Could you check a few things on this model? Use its own coordinates, in mm. Face numbers are marked on the shaded views. A direction names the side the tool comes from. Round coordinates to 2 decimals unless told otherwise and drop trailing zeros. Write each loop counter-clockwise with the first axis right and the second up, starting at its lowest first coordinate (ties: lowest second). Pieces come first, ordered by that corner, then holes. Notation, with made-up numbers: (41, 13.5) - (86, 13.5) arc R7 ccw to (86, 22.5) - close; hole circle Ø9 at (36.25, -29.75). An arc over 180 degrees is marked (long way). Put each result on its own line as item: value.
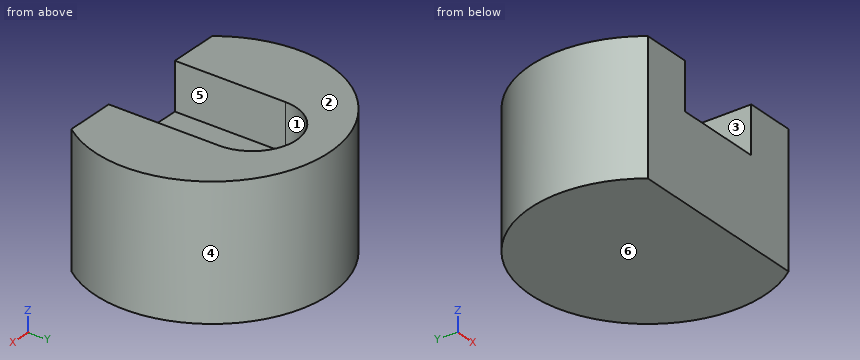
from build123d import *

# Parameters (mm, degrees)
AUFSATZ_LINEAR_AUSTRAGEN1_DEPTH = 5.6
SCHNITT_LINEAR_AUSTRAGEN1_DEPTH = 2


with BuildPart() as part:
    # Skizze1 → Aufsatz-Linear austragen1 (new body)
    with BuildSketch(Plane.XY):
        with BuildLine():
            Line((-4, -3), (4, -3))
            ThreePointArc((4, -3), (0, 5), (-4, -3))
        make_face()
    extrude(amount=-AUFSATZ_LINEAR_AUSTRAGEN1_DEPTH)

    # Skizze2 → Schnitt-Linear austragen1 (cut)
    with BuildSketch(Plane.XY):
        with BuildLine():
            Line((-1.876254768, -1.717667449), (-1.876254768, -3))
            Line((-1.876254768, -3), (1.876254768, -3))
            Line((1.876254768, -3), (1.876254768, -1.717667449))
            Line((1.876254768, -1.717667449), (1.876254768, 1.717667449))
            ThreePointArc((1.876254768, 1.717667449), (0, 3.593922217), (-1.876254768, 1.717667449))
            Line((-1.876254768, 1.717667449), (-1.876254768, -1.717667449))
        make_face()
    extrude(amount=-SCHNITT_LINEAR_AUSTRAGEN1_DEPTH, mode=Mode.SUBTRACT)


solid = part.part
(1) Imagine slicing it at C-C, the plane x = 0. List the corners of the cut face in (y, z) for me.
Values found:
outline: (-3, -5.6) - (5, -5.6) - (5, 0) - (3.59, 0) - (3.59, -2) - (-3, -2) - close
(2) I'm going to push flat-ended pins straight in: pin 1 (1 mm diameter, centred on y = -1, z = -1, fed in from -X); pin 2 (1.1 mm diameter, centred on x = 0, y = 0.5, fed in from +Z); pin 3 (1 mm diameter, centred on y = 4, z = -1, fed in from -X). Where does each tip first touch, or does it pass through?
Values found:
pin 1: stops at x = -4.97
pin 2: stops at z = -2
pin 3: stops at x = -3.57
(3) If we mould it in two halves opening along X, with no side actions, what happens to the marked faces 3, 4, 5 and 6? For each: pulls with the +X half, pulls with the -X half, needs draft (parallel to the pull), parting line crosses it, or undercut.
Values found:
face 3: undercut
face 4: parting line crosses it
face 5: undercut
face 6: needs draft
(4) Imagine slicing it at A-A, the plane y = -2.5. List the corners of the cut face in (x, z) for me, then the cut area to 3 significant figures.
Values found:
outline: (-4.33, -5.6) - (4.33, -5.6) - (4.33, 0) - (1.88, 0) - (1.88, -2) - (-1.88, -2) - (-1.88, 0) - (-4.33, 0) - close
area: 41.0 mm^2
(5) Imagine slicing it at B-B, the plane z = -3.25. List the corners of the cut face in (x, y) for me, then the cut area to 3 significant figures.
Values found:
outline: (-4, -3) - (4, -3) arc R5 ccw (long way) to start
area: 67.4 mm^2
(6) Please list where these lines run through material, in increasing order: probe 1 along X at (y, z) = (0, -1.85); probe 2 along X at (y, z) = (-1.5, -0.5); probe 3 along Y at (x, z) = (3, -4.8). Write a range as from..to.
Values found:
probe 1: x = -5..-1.88, 1.88..5
probe 2: x = -4.77..-1.88, 1.88..4.77
probe 3: y = -3..4
(7) Imagine slicing it at D-D, the plane y = -1. List the corners of the cut face in (x, z) for me, then the cut area to 3 significant figures.
Values found:
outline: (-4.9, -5.6) - (4.9, -5.6) - (4.9, 0) - (1.88, 0) - (1.88, -2) - (-1.88, -2) - (-1.88, 0) - (-4.9, 0) - close
area: 47.4 mm^2
(8) For the marked faces 1 and 2, which set-ups out of +Z, -Z, +X, -X, +Y, -Y let a thin tool reach every point of the face, with its end or its side?
Values found:
face 1: +Z, -Y
face 2: +Z, +X, -X, +Y, -Y
